CAD build for the part. Positions are in the model's coordinates, mm. A direction names the side the tool comes from. Round coordinates to 2 decimals unless told otherwise and drop trailing zeros. Loops run counter-clockwise (first coordinate to the right, second up) from the corner with the lowest first, then second, coordinate; pieces in that order, holes last. Notation, with made-up numbers: (11.5, -37) -> (19.5, -37) arc R37 ccw to (19.5, -1) -> close; hole circle Ø7 at (39, -40). An arc over 180 degrees is marked (long way). Answer as CSV lines item,"result".
```python
from build123d import *

# Parameters (mm, degrees)
F0_W      = 127
F0_H      = 25.4
F0_R      = 6.35
F1_DEPTH  = 12.7
F2_SIZE   = 1.27
F3_W      = 25.4
F3_H      = 6.35
F4_DEPTH  = 25.4
F5_R      = 6.35
F6_DEPTH  = 19.05
F7_DEPTH  = 6.35
F8_SIZE   = 1.27
F9_R      = 6.35
F10_DEPTH = 50.8
F11_SIZE  = 1.27


with BuildPart() as f1:
    # F0 (on Front) → F1 (new body, symmetric)
    with BuildSketch(Plane.XZ):
        with Locations((-63.5, -12.7)):
            Rectangle(F0_W, F0_H)
        with Locations((-95.25, -12.7)):
            Circle(F0_R, mode=Mode.SUBTRACT)
        with Locations((-31.75, -12.7)):
            Circle(F0_R, mode=Mode.SUBTRACT)
    extrude(amount=F1_DEPTH, both=True)

    # F2
    f2_edges = [f1.edges().sort_by_distance(p)[0] for p in [
        (-101.6, -12.7, -12.7),
        (-38.1, -12.7, -12.7),
        (-101.6, 12.7, -12.7),
        (-38.1, 12.7, -12.7),
    ]]
    chamfer(f2_edges, length=F2_SIZE)

    # F3 (on face) → F4 (join)
    with BuildSketch(Plane.YZ):
        with Locations((0, -22.225)):
            Rectangle(F3_W, F3_H)
    extrude(amount=F4_DEPTH)

    # F5 (on face) → F6 (join)
    with BuildSketch(Plane.XY.offset(-19.05)):
        with Locations((12.7, 0)):
            Circle(F5_R)
    extrude(amount=F6_DEPTH)

    # F7 (add): a face of the model
    f7_faces = [f1.faces().sort_by_distance(p)[0] for p in [
        (12.7, 12.3407897552, -19.05),
    ]]
    extrude(f7_faces, amount=F7_DEPTH)

    # F8
    f8_edges = [f1.edges().sort_by_distance(p)[0] for p in [
        (6.35, 0, 0),
    ]]
    chamfer(f8_edges, length=F8_SIZE)

    # F9 (on face) → F10 (join)
    with BuildSketch(Plane.XY):
        with Locations((-15.875, 0)):
            Circle(F9_R)
        with Locations((-47.625, 0)):
            Circle(F9_R)
        with Locations((-79.375, 0)):
            Circle(F9_R)
        with Locations((-111.125, 0)):
            Circle(F9_R)
    extrude(amount=F10_DEPTH)

    # F11
    f11_edges = [f1.edges().sort_by_distance(p)[0] for p in [
        (-22.225, 0, 50.8),
        (-53.975, 0, 50.8),
        (-85.725, 0, 50.8),
        (-117.475, 0, 50.8),
    ]]
    chamfer(f11_edges, length=F11_SIZE)


solid = f1.part
```
Q1. Two-plate mould, pull along X, no slides. Class faces 4 (the cylindrical face through (6.356, 0.279, -7.065)), 5 (the flat face through (13, 0, 0)): pulls with the +X half, pulls with the -X half, needs draft (parallel to the pull), parting line crosses it, or undercut.
Results:
face 4,"undercut"
face 5,"needs draft"
Q2. Slice it at B-B, the plane y = -8.25. Give the cut face in (x, z), and give its area (3 significant figures).
Results:
outline,"(-127, -25.4) -> (25.4, -25.4) -> (25.4, -12.7) -> (0, -12.7) -> (0, 0) -> (-127, 0) -> close; hole circle Ø12.7 at (-95.25, -12.7); hole circle Ø12.7 at (-31.75, -12.7)"
area,"3,300 mm2"
Q3. Slice it at A-A, the plane x = -31.75. Give the cut face in (y, z), and give its area (3 significant figures).
Results:
outline,"(-12.7, -25.4) -> (12.7, -25.4) -> (12.7, -20.32) -> (11.43, -19.05) -> (-11.43, -19.05) -> (-12.7, -20.32) -> close; (-12.7, -5.08) -> (-11.43, -6.35) -> (11.43, -6.35) -> (12.7, -5.08) -> (12.7, 0) -> (-12.7, 0) -> close"
area,"319 mm2"
Q4. Drop flat-ended pins along their axis: pin 1 Ø7.5 at (x, y) = (-94, 2) entering from +Z; pin 2 Ø4 at (y, z) = (7.5, 25) entering from +X; pin 3 Ø2 at (y, z) = (-10, -6.5) entering from +X. Give the stop position or say it passes through.
Results:
pin 1,"z = 0"
pin 2,"x = -12.7"
pin 3,"x = 0"
Q5. Slice it at C-C, the plane z = 10.5. Give the cut face in (x, y) (3 decimals).
Results:
outline,"circle Ø12.7 at (-111.125, 0); circle Ø12.7 at (-79.375, 0); circle Ø12.7 at (-47.625, 0); circle Ø12.7 at (-15.875, 0)"
Q6. Slice it at D-D, the plane y = 2.75. Count the separate pieces of the cut face and the enclosed holes in it, and give its area (3 significant figures).
Results:
separate pieces,"1"
enclosed holes,"2"
area,"5,760 mm2"
Q7. Tool access for faces 1 (the flat face through (-111, 0, 50.8)), 2 (the cylindrical face through (-20.914, -3.864, 24.418)), 3 (the flat face through (0, 0, -6)): list every direction of +Z, -Z, +X, -X, +Y, -Y with a clear straight run to the whole face (end or side of a thin tool).
Results:
face 1,"+Z, +X, -X, +Y, -Y"
face 2,"+Z"
face 3,"+Z, +Y, -Y"
Q8. Probe L1, parallel to X at y = -5, z = 9; L2, parallel to X at y = -3, z = 37; L3, parallel to Z at x = -31.75, y = 3. List the from-to ranges inside material, lowest first. Write a range as [from, to].
Results:
L1,"[-115.04, -107.21], [-83.29, -75.46], [-51.54, -43.71], [-19.79, -11.96]"
L2,"[-116.72, -105.53], [-84.97, -73.78], [-53.22, -42.03], [-21.47, -10.28]"
L3,"[-25.4, -19.05], [-6.35, 0]"
